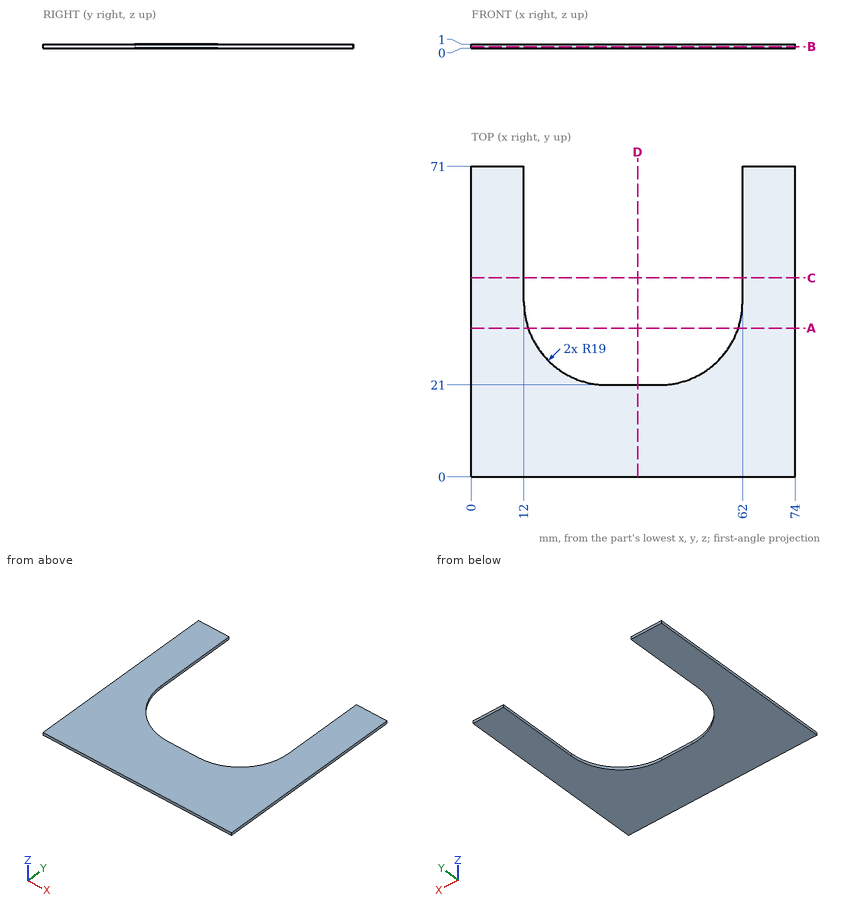
Verification items for this drawing (mm, ordinates from the low corner). Give positions to 0.01 mm unless a question says otherwise; leave off trailing zeros. Loops run counter-clockwise (first coordinate to the right, second up) from the corner with the lowest first, then second, coordinate; pieces in that order, holes last. Notation, with made-up numbers: M 66,38 L 79,38 A29 cw 79,76 Z; hole C -32.5,11.5 d8. An arc over 180 degrees is marked long. Return JSON: item names as keys, results as strings. Group by question number.
1. Cross-section at B-B on z = 0.4. Record the boundary of the cut face in (x, y).
2. Cross-section at D-D on x = 38. Record the boundary of the cut face in (y, z).
3. Cross-section at A-A on y = 34. Record the boundary of the cut face in (x, z), plus the area to 3 significant figures.
4. Cross-section at C-C on y = 45.5. Record the boundary of the cut face in (x, z), plus the area to 3 significant figures.
5. Thickness scan on L1, parallel to X at y = 44.5, z = 0.5; L2, parallel to Y at x = 31, z = 0.8; L3, parallel to X at y = 28.5, z = 0.8. Record the ranges inside material, lowest first.
Return value:
{
 "1": {"outline": "M 0,0 L 74,0 L 74,71 L 62,71 L 62,40 A19 cw 43,21 L 31,21 A19 cw 12,40 L 12,71 L 0,71 Z"},
 "2": {"outline": "M 0,0 L 21,0 L 21,1 L 0,1 Z"},
 "3": {"outline": "M 0,0 L 12.97,0 L 12.97,1 L 0,1 Z; M 61.03,0 L 74,0 L 74,1 L 61.03,1 Z", "area": "25.9 mm^2"},
 "4": {"outline": "M 0,0 L 12,0 L 12,1 L 0,1 Z; M 62,0 L 74,0 L 74,1 L 62,1 Z", "area": "24.0 mm^2"},
 "5": {"L1": "0 to 12, 62 to 74", "L2": "0 to 21", "L3": "0 to 15.88, 58.12 to 74"}
}
